The listing builds one solid part. Answer for the finished solid, in the listing's coordinates (mm). A direction names the side the tool comes from. Give positions to 0.01 mm unless a question says otherwise; leave off trailing zeros. Write each loop counter-clockwise with the first axis right and the second up, starting at its lowest first coordinate (ties: lowest second). Pieces come first, ordered by that corner, then holes. Notation, with made-up numbers: (87, -31) -> (91, -31) arc R24 ccw to (91, -17) -> close; hole circle Ø9 at (76.5, 70.5). An arc over 180 degrees is marked (long way). Put each result on its own line as item: value. Start each with the question number.
1) Find the intervals of material crossed by line 1 along Z through (x, y) = (1.6, 1.5); line 2 along Z through (x, y) = (-0.75, -0.9); line 3 along Y through (x, z) = (0, 14.25), in increasing order. Write a range as from..to.
2) A cutting plane is placed at A-A (y = 0). Write down the section's boundary in (x, z).
3) For a pull along Y with two mould halves and no side action, classify faces 4 (the flat face through (0, 0, 0)), 5 (the flat face through (1.759, 0, 20)), 6 (the cylindrical face through (-3, 0, 19)) as released by +Y, released by -Y, zero draft, split by the parting line, or undercut.
4) Flat-ended cylindrical pins translate along their axes: pin 1 Ø2 at (y, z) = (-1, 3.5) entering from +X; pin 2 Ø3 at (x, z) = (1, 7.5) entering from -Y; pin 3 Ø2 at (y, z) = (0, 7) entering from -X. Find the tip coordinate at first contact, or state that the pin passes through.
5) A cutting plane is placed at B-B (z = 7.5). Write down the section's boundary in (x, y).
6) For faces 1 (the flat face through (1, -2, 20.5)), 2 (the flat face through (1, -2, 18)), 3 (the flat face through (0.89, 1.52, 19.76)), determine the directions among +Z, -Z, +X, -X, +Y, -Y from which every point of the face is accessible in a straight line to the end or side of a thin tool.
from build123d import *

# Parameters (mm, degrees)
SKETCH_1_R          = 2
EXTRUDE_1_DEPTH     = 18
SKETCH_2_R          = 3
EXTRUDE_2_DEPTH     = 2.5
CUT_EXTRUDE_1_DEPTH = 1.5
CHAMFER_1_SIZE      = 0.5
FILLET_1_R          = 0.5


with BuildPart() as part:
    # 草图1 → 凸台-拉伸1 (new body)
    with BuildSketch(Plane.XY):
        Circle(SKETCH_1_R)
    extrude(amount=EXTRUDE_1_DEPTH)

    # 草图2 → 凸台-拉伸2 (add)
    with BuildSketch(Plane.XY.offset(18)):
        Circle(SKETCH_2_R)
    extrude(amount=EXTRUDE_2_DEPTH)

    # 草图4 → 切除-拉伸1 (cut)
    with BuildSketch(Plane.XY.offset(20.5)):
        Polygon((0, 2.031649792), (-1.759460331, 1.015824896), (-1.759460331, -1.015824896), (0, -2.031649792), (1.759460331, -1.015824896), (1.759460331, 1.015824896), align=None)
    extrude(amount=-CUT_EXTRUDE_1_DEPTH, mode=Mode.SUBTRACT)

    # 倒角1
    chamfer_1_edges = [part.edges().sort_by_distance(p)[0] for p in [
        (-2, 0, 0),
    ]]
    chamfer(chamfer_1_edges, length=CHAMFER_1_SIZE)

    # 圆角1
    fillet_1_edges = [part.edges().sort_by_distance(p)[0] for p in [
        (-3, 0, 20.5),
    ]]
    fillet(fillet_1_edges, radius=FILLET_1_R)


solid = part.part
Reply:
1. line 1: z = 18..20.5
1. line 2: z = 0..19
1. line 3: y = -2..2
2. outline: (-3, 18) -> (-2, 18) -> (-2, 0.5) -> (-1.5, 0) -> (1.5, 0) -> (2, 0.5) -> (2, 18) -> (3, 18) -> (3, 20) arc R0.5 ccw to (2.5, 20.5) -> (1.76, 20.5) -> (1.76, 19) -> (-1.76, 19) -> (-1.76, 20.5) -> (-2.5, 20.5) arc R0.5 ccw to (-3, 20) -> close
3. face 4: zero draft
3. face 5: undercut
3. face 6: split by the parting line
4. pin 1: stops at x = 2
4. pin 2: stops at y = -2
4. pin 3: stops at x = -2
5. outline: circle Ø4 at (0, 0)
6. face 1: +Z, +X, -X, +Y, -Y
6. face 2: -Z
6. face 3: +Z
